Design review of the part shown in the three views and the two pictorial views. Dimensions are in mm from the part's minimum x, y and z. A direction names the side the tool comes from. Round coordinates to 2 decimals unless told otherwise and drop trailing zeros. Loops run counter-clockwise (first coordinate to the right, second up) from the corner with the lowest first, then second, coordinate; pieces in that order, holes last. Notation, with made-up numbers: (66, -22) - (75, -22) arc R11 ccw to (75, -7) - close; hole circle Ø4 at (35, 87.5). An arc over 180 degrees is marked (long way). Return JSON: item names as keys, results as strings. Group by question number.
(1) Wall thickness on L1, parallel to X at y = 74.5, z = 73.5; L2, parallel to Y at x = 61, z = 109.5; L3, parallel to Y at x = 61, z = 268: over which ranges is each line inside the solid? List them lowest first. Write a range as [from, to].
(2) We need section A-A, the plane y = 50.8. Write out the cut boundary in (x, z).
(3) We need section D-D, the plane x = 30.5. Write out the cut boundary in (y, z).
(4) The part is to be moulded in two halves that separate along X. For the marked faces 3, 4 and 5, say which applies: pulls with the +X half, pulls with the -X half, needs draft (parallel to the pull), parting line crosses it, or undercut.
(5) Clearance check with flat-ended pins moving along their axes: pin 1 (1 mm diameter, centred on x = 62.5, z = 138.5, fed in from -Y); pin 2 (3 mm diameter, centred on x = 23.5, z = 247.5, fed in from -Y); pin 3 (2 mm diameter, centred on x = 65.5, y = 73.5, fed in from +Z). State where each tip first meets the part, or that it passes through.
(6) For the marked faces 1 and 2, list the 3-axis set-ups (+Z, -Z, +X, -X, +Y, -Y) from which the entire face can be reached by the end or side of a thin tool; tool diameter is ignored.
(7) We need section B-B, the plane z = 199.5. Write out the cut boundary in (x, y), and give its area (3 significant figures).
(8) We need section C-C, the plane x = 57. Write out the cut boundary in (y, z), and give its area (3 significant figures).
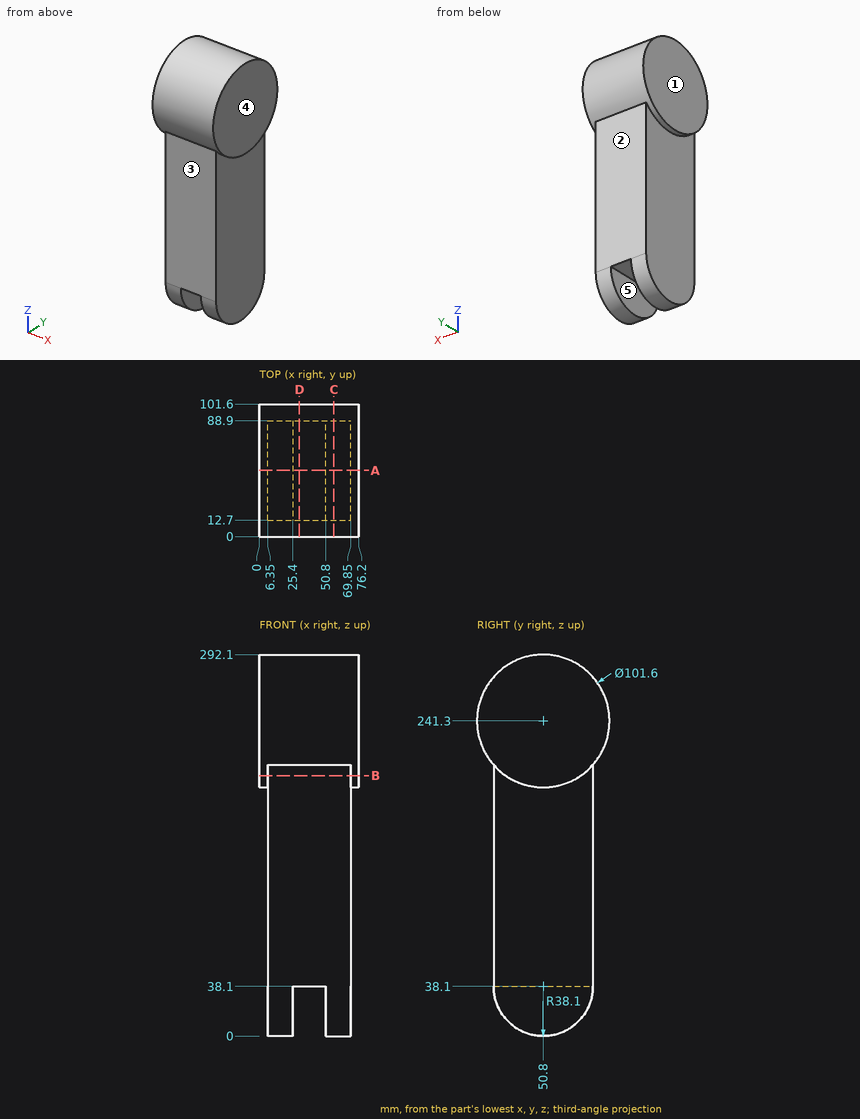
Solutions:
{
 "1": {"L1": "[6.35, 69.85]", "L2": "[12.7, 88.9]", "L3": "[7.58, 94.02]"},
 "2": {"outline": "(0, 190.5) - (6.35, 190.5) - (6.35, 0) - (25.4, 0) - (25.4, 38.1) - (50.8, 38.1) - (50.8, 0) - (69.85, 0) - (69.85, 190.5) - (76.2, 190.5) - (76.2, 292.1) - (0, 292.1) - close"},
 "3": {"outline": "(12.7, 38.1) - (88.9, 38.1) - (88.9, 207.7) arc R50.8 ccw (long way) to (12.7, 207.7) - close"},
 "4": {"face 3": "needs draft", "face 4": "pulls with the +X half", "face 5": "undercut"},
 "5": {"pin 1": "y = 12.7", "pin 2": "y = 0.22", "pin 3": "z = 287.23"},
 "6": {"face 1": "+Z, -Z, -X, +Y, -Y", "face 2": "-Z, +X, -X, +Y"},
 "7": {"outline": "(0, 21.93) - (6.35, 21.93) - (6.35, 12.7) - (69.85, 12.7) - (69.85, 21.93) - (76.2, 21.93) - (76.2, 79.67) - (69.85, 79.67) - (69.85, 88.9) - (6.35, 88.9) - (6.35, 79.67) - (0, 79.67) - close", "area": "5,570 mm^2"},
 "8": {"outline": "(12.7, 38.1) arc R38.1 ccw to (88.9, 38.1) - (88.9, 207.7) arc R50.8 ccw (long way) to (12.7, 207.7) - close", "area": "22,400 mm^2"}
}
